The listing builds one solid part. Answer for the finished solid, in the listing's coordinates (mm). Face numbers are marked on the shaded views. A direction names the side the tool comes from. Give positions to 0.01 mm unless a question says otherwise; leave off trailing zeros. Order: outer loops, then holes, each group sorted by start corner. A loop starts at its lowest first (then second) coordinate and runs counter-clockwise, first axis right, second up. Notation, with made-up numbers: (82.25, 63.25) - (116.25, 63.25) arc R33 ccw to (116.25, 101.25) - close; hole circle Ø10 at (10.5, 56). An arc over 180 degrees is marked (long way). Write each question's results on one line, items separated by ' | '. Start each with the question number.
1. Section A-A (y = 16) is taken. State how many separate pieces and enclosed holes the cut face has, and give its area (3 significant figures).
2. Section B-B (x = 82) is taken. Give the vertices of the cut face in (y, z), and give its area (3 significant figures).
3. Find the intervals of material crossed by L1, parallel to X at y = 5.5, z = 4; L2, parallel to Y at x = 6, z = 4.75; L3, parallel to X at y = 43, z = 6.75, in increasing order.
4. Which of the six approach directions +Z, -Z, +X, -X, +Y, -Y give full straight-line access (tool end or side, diameter ignored) to the marked faces 1, 2 and 3?
5. Section D-D (x = 22) is taken. Give the vertices of the cut face in (y, z), and give its area (3 significant figures).
6. Determine the mould class of the marked faces 4, 5 and 6 for opening direction Y: released by +Y, released by -Y, zero draft, split by the parting line, or undercut.
7. Flat-ended cylindrical pins translate along their axes: pin 1 (3 mm diameter, centred on x = 92, y = 6, fed in from -Z); pin 2 (16 mm diameter, centred on x = 49, y = 16, fed in from -Z); pin 3 (1.5 mm diameter, centred on x = 55.5, y = 40, fed in from +Z); pin 4 (0.8 mm diameter, centred on x = 91.5, z = -5.5, fed in from -Y). Find the tip coordinate at first contact, or state that the pin passes through.
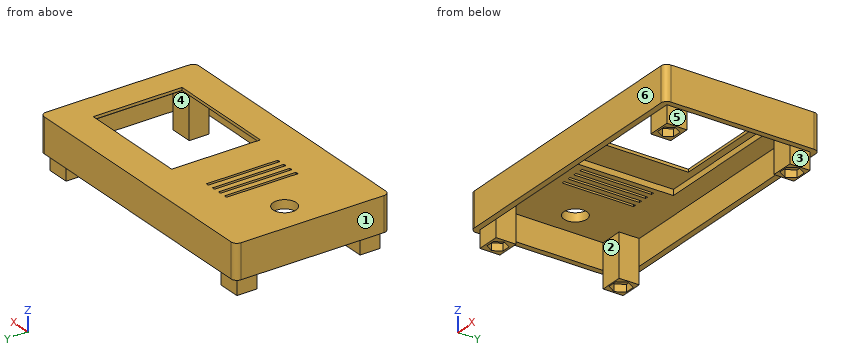
from build123d import *

# Parameters (mm, degrees)
SKETCH_W        = 97
SKETCH_H        = 54
SKETCH_R        = 4
SKETCH_W_2      = 39
SKETCH_H_2      = 31
PAD_DEPTH       = 12
SKETCH001_W     = 93
SKETCH001_H     = 50
POCKET_DEPTH    = 9
SKETCH002_W     = 53
SKETCH002_H     = 36
POCKET001_DEPTH = 2
SKETCH003_W     = 1
SKETCH003_H     = 25
POCKET002_DEPTH = 12.001
FILLET_R        = 2
SKETCH004_W     = 8
SKETCH004_H     = 7
SKETCH004_R     = 1.7
PAD001_DEPTH    = 15
POCKET003_DEPTH = 2.5
POCKET004_DEPTH = 2.5
POCKET005_DEPTH = 2.5
POCKET006_DEPTH = 2.5


with BuildPart() as part:
    # Sketch → Pad (new body)
    with BuildSketch(Plane.XY):
        with Locations((48.5, 27)):
            Rectangle(SKETCH_W, SKETCH_H)
        with Locations((11, 29)):
            Circle(SKETCH_R, mode=Mode.SUBTRACT)
        with Locations((67.5, 27)):
            Rectangle(SKETCH_W_2, SKETCH_H_2, mode=Mode.SUBTRACT)
    extrude(amount=PAD_DEPTH)

    # Sketch001 → Pocket (cut)
    with BuildSketch(Plane(origin=(0, 0, 0), x_dir=(1, 0, 0), z_dir=(0, 0, -1))):
        with Locations((48.5, -27)):
            Rectangle(SKETCH001_W, SKETCH001_H)
    extrude(amount=-POCKET_DEPTH, mode=Mode.SUBTRACT)

    # Sketch002 → Pocket001 (cut)
    with BuildSketch(Plane(origin=(0, 0, 9), x_dir=(1, 0, 0), z_dir=(0, 0, -1))):
        with Locations((63.5, -27)):
            Rectangle(SKETCH002_W, SKETCH002_H)
    extrude(amount=-POCKET001_DEPTH, mode=Mode.SUBTRACT)

    # Sketch003 → Pocket002 (cut, through all)
    with BuildSketch(Plane.XY.offset(12)):
        with Locations((28.5, 27)):
            Rectangle(SKETCH003_W, SKETCH003_H)
        with Locations((31.5, 27)):
            Rectangle(SKETCH003_W, SKETCH003_H)
        with Locations((25.5, 27)):
            Rectangle(SKETCH003_W, SKETCH003_H)
        with Locations((34.5, 27)):
            Rectangle(SKETCH003_W, SKETCH003_H)
    extrude(amount=-POCKET002_DEPTH, mode=Mode.SUBTRACT)

    # Fillet
    fillet_edges = [part.edges().sort_by_distance(p)[0] for p in [
        (97, 0, 6),
        (0, 0, 6),
        (97, 54, 6),
        (0, 54, 6),
    ]]
    fillet(fillet_edges, radius=FILLET_R)

    # Sketch004 → Pad001 (new body)
    with BuildSketch(Plane(origin=(0, 0, 9), x_dir=(1, 0, 0), z_dir=(0, 0, -1))):
        with Locations((6, -5.5)):
            Rectangle(SKETCH004_W, SKETCH004_H)
        with Locations((6, -5.5)):
            Circle(SKETCH004_R, mode=Mode.SUBTRACT)
        with Locations((91, -5.5)):
            Rectangle(SKETCH004_W, SKETCH004_H)
        with Locations((91, -5.5)):
            Circle(SKETCH004_R, mode=Mode.SUBTRACT)
        with Locations((6, -48.5)):
            Rectangle(SKETCH004_W, SKETCH004_H)
        with Locations((6, -48.5)):
            Circle(SKETCH004_R, mode=Mode.SUBTRACT)
        with Locations((91, -48.5)):
            Rectangle(SKETCH004_W, SKETCH004_H)
        with Locations((91, -48.5)):
            Circle(SKETCH004_R, mode=Mode.SUBTRACT)
    extrude(amount=PAD001_DEPTH)

    # Sketch006 → Pocket003 (cut)
    with BuildSketch(Plane(origin=(0, 0, -6), x_dir=(1, 0, 0), z_dir=(0, 0, -1))):
        Polygon((7.6, -8.271281), (9.2, -5.5), (7.6, -2.728719), (4.4, -2.728719), (2.8, -5.5), (4.4, -8.271281), align=None)
    extrude(amount=-POCKET003_DEPTH, mode=Mode.SUBTRACT)

    # Sketch007 → Pocket004 (cut)
    with BuildSketch(Plane(origin=(0, 0, -6), x_dir=(1, 0, 0), z_dir=(0, 0, -1))):
        Polygon((92.6, -8.271281), (94.2, -5.5), (92.6, -2.728719), (89.4, -2.728719), (87.8, -5.5), (89.4, -8.271281), align=None)
    extrude(amount=-POCKET004_DEPTH, mode=Mode.SUBTRACT)

    # Sketch008 → Pocket005 (cut)
    with BuildSketch(Plane(origin=(0, 0, -6), x_dir=(1, 0, 0), z_dir=(0, 0, -1))):
        Polygon((7.75, -51.531089), (9.5, -48.5), (7.75, -45.468911), (4.25, -45.468911), (2.5, -48.5), (4.25, -51.531089), align=None)
    extrude(amount=-POCKET005_DEPTH, mode=Mode.SUBTRACT)

    # Sketch010 → Pocket006 (cut)
    with BuildSketch(Plane(origin=(0, 0, -6), x_dir=(1, 0, 0), z_dir=(0, 0, -1))):
        Polygon((92.75, -51.531089), (94.5, -48.5), (92.75, -45.468911), (89.25, -45.468911), (87.5, -48.5), (89.25, -51.531089), align=None)
    extrude(amount=-POCKET006_DEPTH, mode=Mode.SUBTRACT)


solid = part.part
Reported:
1) separate pieces: 6 | enclosed holes: 0 | area: 170 mm²
2) outline: (0, 0) - (2, 0) - (2, 9) - (9, 9) - (9, 11) - (11.5, 11) - (11.5, 12) - (0, 12) - close; (42.5, 11) - (45, 11) - (45, 9) - (52, 9) - (52, 0) - (54, 0) - (54, 12) - (42.5, 12) - close | area: 95.0 mm²
3) L1: 0 to 4.3, 7.7 to 10, 87 to 89.3, 92.7 to 97 | L2: 0 to 3.8, 7.2 to 9, 45 to 46.8, 50.2 to 54 | L3: 0 to 2, 95 to 97
4) face 1: +Z, -Z, -X, +Y, -Y | face 2: -Z | face 3: -Z, +X, +Y, -Y
5) outline: (0, 0) - (2, 0) - (2, 9) - (52, 9) - (52, 0) - (54, 0) - (54, 12) - (0, 12) - close | area: 198 mm²
6) face 4: undercut | face 5: zero draft | face 6: released by -Y
7) pin 1: z = -3.5 | pin 2: z = 9 | pin 3: through | pin 4: y = 2
